Model file for the job. Use its own axes, mm. A direction names the side the tool comes from. Coordinates: 2 decimals unless noted, no trailing zeros. Write each loop counter-clockwise with the first axis right and the second up, starting at its lowest first coordinate (ties: lowest second). Pieces come first, ordered by that corner, then holes. Notation, with made-up numbers: (29.25, 68.25) - (56.25, 68.25) arc R6 cw to (56.25, 77.25) - close; hole circle Ø8 at (65.5, 25). An arc over 180 degrees is marked (long way). Put each result on its own line as item: value. Start each with the question number.
1. Saw through at A-A, the plane z = 0. Write the cut outline in (x, y).
2. Drop flat-ended pins along their axis: P1, Ø6, axis at x = -18.5, z = -10.5, coming from the +Y side; P2, Ø2.5, axis at x = -27, y = 4, coming from the -Z side; P3, Ø1.5, axis at y = 3, z = 26, coming from the -X side. Give the stop position or say it passes through.
3. Pull direction Z, two halves, no side cores. Call faces 6 (the face through (27, 2.54, -27.07)), 7 (the face through (-26, 5, 0)), 8 (the face through (13.814, 1.014, 25.221)): released by +Z, released by -Z, zero draft, split by the parting line, or undercut.
4. Saw through at C-C, the plane x = 10. Write the cut outline in (y, z).
5. Saw through at D-D, the plane z = 15.5. Write the cut outline in (x, y), plus the area to 3 significant figures.
6. Saw through at B-B, the plane y = 3.7. Give the number of separate pieces and of enclosed holes in the cut face, plus the area to 3 significant figures.
7. Drill centre lines: L1, parallel to X at y = 0.4, z = 15.5; L2, parallel to Z at x = 24.5, y = 1.85; L3, parallel to Z at x = -25, y = 1.5. Where is each one in solid material? Low to high. Write a range as from..to.
8. Which spindle directions (+Z, -Z, +X, -X, +Y, -Y) get a long thin tool onto all of the face, cutting with end or side? Do faces 1 (the face through (27, 4, -18.5)), 2 (the face through (-27, 4, 18.5)), 3 (the face through (-18.5, 4, -27)), 4 (the face through (0, 0, -26)), 5 (the face through (22.4, 2, -7.6)). Say none if no direction does.
```python
from build123d import *

# Parameters (mm, degrees)
SKETCH1_W           = 57
SKETCH1_H           = 57
SKETCH1_R           = 25.1
BOSS_EXTRUDE1_DEPTH = 5
SKETCH1_3_R         = 25.1
SKETCH1_3_R_2       = 23.5
BOSS_EXTRUDE2_DEPTH = 2
FILLET1_R           = 5
SKETCH2_R           = 2.5
SKETCH2_R_2         = 1.7
CUT_EXTRUDE2_DEPTH  = 41.614036982
SKETCH3_R           = 1.7
CUT_EXTRUDE3_DEPTH  = 3
CUT_EXTRUDE4_DEPTH  = 1.1
CIRPATTERN1_COUNT   = 4


with BuildPart() as part:
    # Sketch1 → Boss-Extrude1 (new body)
    with BuildSketch(Plane(origin=(0, 0, 0), x_dir=(1, 0, 0), z_dir=(0, 1, 0))):
        Rectangle(SKETCH1_W, SKETCH1_H)
        with Locations(Location((0, 0, 0), (0, 0, 270))):
            Circle(SKETCH1_R, mode=Mode.SUBTRACT)
    extrude(amount=BOSS_EXTRUDE1_DEPTH)

    # Sketch1_3 → Boss-Extrude2 (add)
    with BuildSketch(Plane(origin=(0, 0, 0), x_dir=(1, 0, 0), z_dir=(0, 1, 0))):
        with Locations(Location((0, 0, 0), (0, 0, 270))):
            Circle(SKETCH1_3_R)
        with Locations(Location((0, 0, 0), (0, 0, 270))):
            Circle(SKETCH1_3_R_2, mode=Mode.SUBTRACT)
    extrude(amount=BOSS_EXTRUDE2_DEPTH)

    # Fillet1
    fillet1_edges = [part.edges().sort_by_distance(p)[0] for p in [
        (-28.5, 2.5, -28.5),
        (28.5, 2.5, -28.5),
        (28.5, 2.5, 28.5),
        (-28.5, 2.5, 28.5),
    ]]
    fillet(fillet1_edges, radius=FILLET1_R)

    # Sketch2 → Cut-Extrude2 (cut, through all)
    with BuildSketch(Plane(origin=(0, 5, 0), x_dir=(1, 0, 0), z_dir=(0, 1, 0))):
        with Locations(Location((-23.5, 23.5, 0), (0, 0, 270))):
            Circle(SKETCH2_R)
        with Locations(Location((-15.5, 25, 0), (0, 0, 270))):
            Circle(SKETCH2_R_2)
    cut_extrude2 = extrude(amount=-CUT_EXTRUDE2_DEPTH, mode=Mode.SUBTRACT)

    # Sketch3 → Cut-Extrude3 (cut)
    with BuildSketch(Plane(origin=(0, 5, 0), x_dir=(1, 0, 0), z_dir=(0, 1, 0))):
        with BuildLine():
            ThreePointArc((-18.5, 25), (-15.451669698, 22.000389328), (-12.501557212, 25.09664806))
            Line((-12.501557212, 25.09664806), (-12.611256608, 28.5))
            Line((-12.611256608, 28.5), (-18.5, 28.5))
            Line((-18.5, 28.5), (-18.5, 25))
        make_face()
        with Locations(Location((-15.5, 25, 0), (0, 0, 270))):
            Circle(SKETCH3_R, mode=Mode.SUBTRACT)
    cut_extrude3 = extrude(amount=-CUT_EXTRUDE3_DEPTH, mode=Mode.SUBTRACT)

    # Sketch4 → Cut-Extrude4 (cut)
    with BuildSketch(Plane.XZ):
        Polygon((-27.5, -11), (-27.5, 11), (-28.5, 12), (-28.5, -12), align=None)
    cut_extrude4 = extrude(amount=-CUT_EXTRUDE4_DEPTH, mode=Mode.SUBTRACT)

    # CirPattern1: Cut-Extrude2, Cut-Extrude3, Cut-Extrude4 ×4 about axis
    cirpattern1_axis = Axis((0, 0, 0), (0, 1, 0))
    add([cut_extrude2.rotate(cirpattern1_axis, i * 360 / CIRPATTERN1_COUNT) for i in range(1, CIRPATTERN1_COUNT)], mode=Mode.SUBTRACT)
    add([cut_extrude3.rotate(cirpattern1_axis, i * 360 / CIRPATTERN1_COUNT) for i in range(1, CIRPATTERN1_COUNT)], mode=Mode.SUBTRACT)
    add([cut_extrude4.rotate(cirpattern1_axis, i * 360 / CIRPATTERN1_COUNT) for i in range(1, CIRPATTERN1_COUNT)], mode=Mode.SUBTRACT)


solid = part.part
```
Final values:
1. outline: (-28.5, 1.1) - (-27.5, 1.1) - (-27.5, 0) - (-23.5, 0) - (-23.5, 2) - (-25.1, 2) - (-25.1, 5) - (-28.5, 5) - close; (23.5, 0) - (27.5, 0) - (27.5, 1.1) - (28.5, 1.1) - (28.5, 5) - (25.1, 5) - (25.1, 2) - (23.5, 2) - close
2. P1: stops at y = 2
2. P2: stops at z = -27.97
2. P3: stops at x = -28.18
3. face 6: released by -Z
3. face 7: zero draft
3. face 8: undercut
4. outline: (0, -27.5) - (1.1, -27.5) - (1.1, -28.5) - (5, -28.5) - (5, -23.02) - (2, -23.02) - (2, -21.27) - (0, -21.27) - close; (0, 21.27) - (2, 21.27) - (2, 23.02) - (5, 23.02) - (5, 28.5) - (1.1, 28.5) - (1.1, 27.5) - (0, 27.5) - close
5. outline: (-28.5, 0) - (-26.7, 0) - (-26.7, 2) - (-28.5, 2) - close; (-23.3, 0) - (-17.66, 0) - (-17.66, 2) - (-19.74, 2) - (-19.74, 5) - (-22, 5) - (-22, 2) - (-23.3, 2) - close; (17.66, 0) - (28.5, 0) - (28.5, 5) - (19.74, 5) - (19.74, 2) - (17.66, 2) - close
5. area: 69.6 mm²
6. separate pieces: 1
6. enclosed holes: 5
6. area: 1,030 mm²
7. L1: x = -28.5..-26.7, -23.3..-17.66, 17.66..28.5
7. L2: z = -28.4..-25.79, -21.21..-17.12, -13.88..21.21, 25.79..28.4
7. L3: z = -28.27..-25.5, -21.5..13.8, 17.2..21.5, 25.5..28.27
8. face 1: +X, +Y
8. face 2: -X, +Y
8. face 3: -Z, +Y
8. face 4: +Z, -Z, +X, -X, -Y
8. face 5: +Y
